Build history of the part. All positions in model axes, mm. Face numbers are marked on the shaded views. A direction names the side the tool comes from. Round coordinates to 2 decimals unless told otherwise and drop trailing zeros. Write each loop counter-clockwise with the first axis right and the second up, starting at its lowest first coordinate (ties: lowest second). Pieces come first, ordered by that corner, then holes. Notation, with made-up numbers: M 54,-18 L 73,-18 A26 cw 73,0 Z; hole C 45.25,-38 d11. An arc over 180 degrees is marked long. Use a Markdown table: item, result.
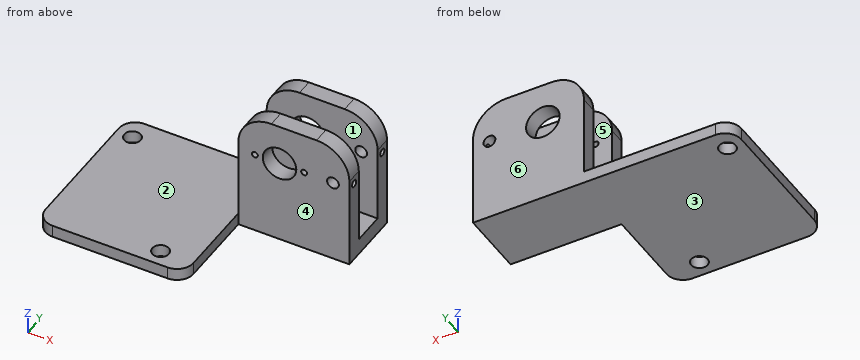
from build123d import *

# Parameters (mm, degrees)
F0_R     = 6.477
F0_R_2   = 2.286
F1_DEPTH = 25.4
F2_W     = 12.7
F2_H     = 54.030560414
F3_DEPTH = 42.8635
F4_R     = 3.175
F5_DEPTH = 4.7625
F6_R     = 1.143
F7_DEPTH = 6.35
F8_R     = 1.397
F9_DEPTH = 4.5415286302


with BuildPart() as f1:
    # F0 (on Front) → F1 (new body)
    with BuildSketch(Plane.XZ):
        with BuildLine():
            Line((-15.875, 35.8775), (-15.875, 0))
            Line((-15.875, 0), (26.9875, 0))
            Line((26.9875, 0), (26.9875, 35.8775))
            ThreePointArc((26.9875, 35.8775), (23.2677561211, 44.8577561211), (14.2875, 48.5775))
            Line((14.2875, 48.5775), (-3.175, 48.5775))
            ThreePointArc((-3.175, 48.5775), (-12.1552561211, 44.8577561211), (-15.875, 35.8775))
        make_face()
        with Locations((0, 32.7025)):
            Circle(F0_R, mode=Mode.SUBTRACT)
        with Locations((20.6375, 32.7025)):
            Circle(F0_R_2, mode=Mode.SUBTRACT)
    extrude(amount=F1_DEPTH)

    # F2 (on face) → F3 (cut, through all)
    with BuildSketch(Plane(origin=(-15.875, 0, 0), x_dir=(0, -1, 0), z_dir=(-1, 0, 0))):
        with Locations((12.7, 33.365280207)):
            Rectangle(F2_W, F2_H)
    extrude(amount=-F3_DEPTH, mode=Mode.SUBTRACT)

    # F4 (on Top) → F5 (join)
    with BuildSketch(Plane.XY):
        with BuildLine():
            Line((-15.875, -55.753), (-15.875, 0))
            Line((-15.875, 0), (-66.675, 0))
            ThreePointArc((-66.675, 0), (-71.1651280605, -1.8598719395), (-73.025, -6.35))
            Line((-73.025, -6.35), (-73.025, -55.753))
            ThreePointArc((-73.025, -55.753), (-71.1651280605, -60.2431280605), (-66.675, -62.103))
            Line((-66.675, -62.103), (-22.225, -62.103))
            ThreePointArc((-22.225, -62.103), (-17.7348719395, -60.2431280605), (-15.875, -55.753))
        make_face()
        with Locations((-28.575, -55.753)):
            Circle(F4_R, mode=Mode.SUBTRACT)
        with Locations((-66.675, -8.128)):
            Circle(F4_R, mode=Mode.SUBTRACT)
    extrude(amount=F5_DEPTH)

    # F6 (on face) → F7 (cut, through all)
    with BuildSketch(Plane.XZ.offset(25.4)):
        with Locations((9.525, 32.7025)):
            Circle(F6_R)
        with Locations((-9.525, 32.7025)):
            Circle(F6_R)
    extrude(amount=-F7_DEPTH, mode=Mode.SUBTRACT)

    # F8 (on face) → F9 (cut, through all)
    with BuildSketch(Plane.YZ.offset(26.9875)):
        with Locations((-22.225, 32.7025)):
            Circle(F8_R)
        with Locations((-3.175, 32.7025)):
            Circle(F8_R)
    extrude(amount=-F9_DEPTH, mode=Mode.SUBTRACT)


solid = f1.part
Q1. Drop flat-ended pins along their axis: P1, Ø12.5, axis at y = -15, z = 19, coming from the -X side (3 decimals); P2, Ø1.4, axis at y = -48, z = 1.5, coming from the +X side (3 decimals); P3, Ø2, axis at x = 9.52, z = 32.7, coming from the -Y side. Give the stop position or say it passes through.
Response values:
| item | result |
|---|---|
| P1 | stops at x = -15.875 |
| P2 | stops at x = -15.875 |
| P3 | stops at y = -6.35 |
Q2. Cut at C-C on x = -30. Give the cut face in (y, z).
Response values:
| item | result |
|---|---|
| outline | M -62.1,0 L -58.59,0 L -58.59,4.76 L -62.1,4.76 Z; M -52.92,0 L 0,0 L 0,4.76 L -52.92,4.76 Z |
Q3. Two-plate mould, pull along Y, no slides. Class the marked faces 4, 5 and 6: +Y half, -Y half, draft (parallel to the pull), parting line (faces both ways), or undercut.
Response values:
| item | result |
|---|---|
| face 4 | -Y half |
| face 5 | undercut |
| face 6 | +Y half |
Q4. Cut at A-A on x = 0. Give the cut face in (y, z).
Response values:
| item | result |
|---|---|
| outline | M -25.4,0 L 0,0 L 0,26.23 L -6.35,26.23 L -6.35,6.35 L -19.05,6.35 L -19.05,26.23 L -25.4,26.23 Z; M -25.4,39.18 L -19.05,39.18 L -19.05,48.58 L -25.4,48.58 Z; M -6.35,39.18 L 0,39.18 L 0,48.58 L -6.35,48.58 Z |
Q5. Which spindle directions (+Z, -Z, +X, -X, +Y, -Y) get a long thin tool onto all of the face, cutting with end or side? Do the marked faces 1, 2 and 3. Say none if no direction does.
Response values:
| item | result |
|---|---|
| face 1 | +Z, +X, -X |
| face 2 | +Z, -X, +Y, -Y |
| face 3 | -Z, +X, -X, +Y, -Y |
Q6. Cut at D-D on y = -22. Give the cut face in (x, z) (1 decimal).
Response values:
| item | result |
|---|---|
| outline | M -73,0 L 27,0 L 27,31.3 L 22.5,31.3 A2.3 cw long 22.5,34.1 L 27,34.1 L 27,35.9 A12.7 ccw 14.3,48.6 L -3.2,48.6 A12.7 ccw -15.9,35.9 L -15.9,4.8 L -73,4.8 Z; hole C -9.5,32.7 d2.3; hole C 0,32.7 d13; hole C 9.5,32.7 d2.3 |
Q7. Drill centre lines: L1, parallel to Y at x = -2.5, z = 46.5; L2, parallel to Z at x = 0, y = -4; L3, parallel to Z at x = 11, y = -12. Where is each one in solid material? Low to high.
Response values:
| item | result |
|---|---|
| L1 | y = -25.4 to -19.05, -6.35 to 0 |
| L2 | z = 0 to 26.23, 39.18 to 48.58 |
| L3 | z = 0 to 6.35 |
